from build123d import *

# Parameters (mm, degrees)
SKETCH_2_R               = 12
EXTRUDE_1_DEPTH          = 8
SKETCH_3_R               = 12
SKETCH_3_R_2             = 10
CUT_EXTRUDE_1_DEPTH      = 5
CUT_EXTRUDE_2_DEPTH      = 19.761663039
CUT_EXTRUDE_2_DEPTH_BACK = 19.761663039
SKETCH_4_R               = 2


with BuildPart() as part:
    # 草图2 → 凸台-拉伸1 (new, symmetric)
    with BuildSketch(Plane(origin=(0, 0, 0), x_dir=(0, 0, -1), z_dir=(1, 0, 0))):
        Circle(SKETCH_2_R)
    extrude(amount=EXTRUDE_1_DEPTH, both=True)

    # 草图3 → 切除-拉伸1 (cut, symmetric)
    with BuildSketch(Plane(origin=(0, 0, 0), x_dir=(0, 0, -1), z_dir=(1, 0, 0))):
        Circle(SKETCH_3_R)
        Circle(SKETCH_3_R_2, mode=Mode.SUBTRACT)
    extrude(amount=CUT_EXTRUDE_1_DEPTH, both=True, mode=Mode.SUBTRACT)

    # 草图4 → 切除-拉伸2 (cut, two sides: drawn at the far end of the back side and taken through both)
    with BuildSketch(Plane(origin=(0, 0, 0), x_dir=(0, 0, -1), z_dir=(1, 0, 0)).offset(-CUT_EXTRUDE_2_DEPTH_BACK)):
        Circle(SKETCH_4_R)
    extrude(amount=CUT_EXTRUDE_2_DEPTH + CUT_EXTRUDE_2_DEPTH_BACK, mode=Mode.SUBTRACT)


solid = part.part
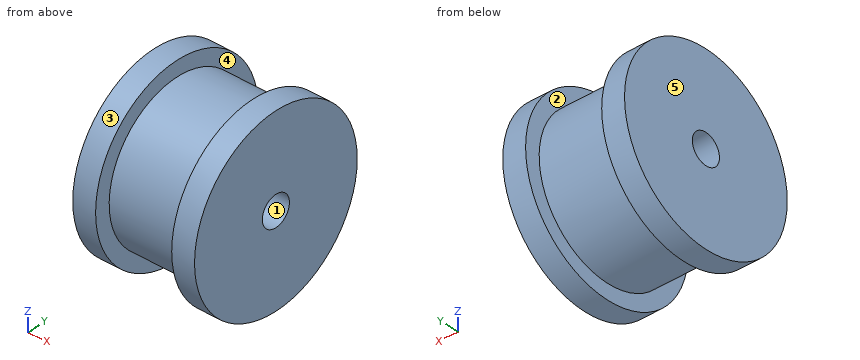
The listing builds one solid part. Answer for the finished solid, in the listing's coordinates (mm). Face numbers are marked on the shaded views. A direction names the side the tool comes from. Coordinates: 2 decimals unless noted, no trailing zeros. Order: outer loops, then holes, each group sorted by start corner. A loop starts at its lowest first (then second) coordinate and runs counter-clockwise, first axis right, second up.
Q1. A cutting plane is placed at D-D, the plane z = -5. Write down the section's boundary in (x, y), and give its area (3 significant figures).
Q2. Consider line 1 (X direction, y = 10.5, z = 0); line 2 (Y direction, x = -0.5, z = 0); line 3 (Z direction, x = -4.5, y = -1.25). Determine where each line is inside the solid, lowest interval first.
Q3. Which of the six approach directions +Z, -Z, +X, -X, +Y, -Y give full straight-line access (tool end or side, diameter ignored) to the marked faces 4 and 5?
Q4. For a pull along Y with two mould halves and no side action, classify the marked faces 1, 2 and 3 as pulls with the +Y half, pulls with the -Y half, needs draft (parallel to the pull), parting line crosses it, or undercut.
Q5. Given P1, Ø1.5, axis at x = -4, z = 3.5, coming from the -Y side; P2, Ø1, axis at x = 6.5, z = -9, coming from the -Y side; P3, Ø1.5, axis at x = -4, z = -4, coming from the +Y side, each flat-ended and moving along its own axis, determine where each tip first touches the part or whether it passes through.
Q6. A cutting plane is placed at A-A, the plane y = 0. Write down the section's boundary in (x, z), and give its area (3 significant figures).
Q7. A cutting plane is placed at C-C, the plane x = 3. Write down the section's boundary in (y, z), and give its area (3 significant figures).
Answers follow:
1. outline: (-8, -10.91) - (-5, -10.91) - (-5, -8.66) - (5, -8.66) - (5, -10.91) - (8, -10.91) - (8, 10.91) - (5, 10.91) - (5, 8.66) - (-5, 8.66) - (-5, 10.91) - (-8, 10.91) - close
1. area: 304 mm2
2. line 1: x = -8 to -5, 5 to 8
2. line 2: y = -10 to -2, 2 to 10
2. line 3: z = -9.92 to -1.56, 1.56 to 9.92
3. face 4: none
3. face 5: +Z, -Z, -X, +Y, -Y
4. face 1: undercut
4. face 2: needs draft
4. face 3: parting line crosses it
5. P1: stops at y = -9.61
5. P2: stops at y = -8.47
5. P3: stops at y = 9.46
6. outline: (-8, -12) - (-5, -12) - (-5, -10) - (5, -10) - (5, -12) - (8, -12) - (8, -2) - (-8, -2) - close; (-8, 2) - (8, 2) - (8, 12) - (5, 12) - (5, 10) - (-5, 10) - (-5, 12) - (-8, 12) - close
6. area: 280 mm2
7. outline: circle Ø20 at (0, 0); hole circle Ø4 at (0, 0)
7. area: 302 mm2
